Job drawing, mm, ordinate dimensions from the low corner. One solid piece. A direction names the side the tool comes from. Coordinates: 2 decimals unless noted, no trailing zeros. Write each loop counter-clockwise with the first axis right and the second up, starting at its lowest first coordinate (ties: lowest second). Pieces come first, ordered by that corner, then holes. Notation, with made-up numbers: (44, 81) -> (87, 81) arc R3 ccw to (87, 85) -> close; hole circle Ø5 at (62.5, -3.5). An arc over 180 degrees is marked (long way). One line per question, with ' | ' between items. Start each with the question number.
Item 1: 3-axis set-ups, long thin cutter, end or side, ignore diameter. For the marked faces 1 and 2: which of +Z, -Z, +X, -X, +Y, -Y reach the whole face in a straight line?
Item 2: Saw through at D-D (y = 4.5). List the corners of the cut face in (x, z).
Item 3: Pin check, flat tips, straight feed: pin 1 (1 mm diameter, centred on x = 17.5, z = 0.5, fed in from +Y); pin 2 (4 mm diameter, centred on x = 11, y = 8, fed in from +Z); pin 3 (1.7 mm diameter, centred on x = 11.25, y = 19.75, fed in from +Z). Stop position of each tip, or through.
Item 4: Two-plate mould, pull along Y, no slides. Class the marked faces 3, 4 and 5: pulls with the +Y half, pulls with the -Y half, needs draft (parallel to the pull), parting line crosses it, or undercut.
Item 5: Probe probe 1 along Y at (x, z) = (11.25, 1.2) (1 decimal); probe 2 along Y at (x, z) = (12.5, 1.65) (1 decimal); probe 3 along Z at (x, y) = (10.5, 11.75). List the from-to ranges inside material, lowest first. Write a range as [from, to].
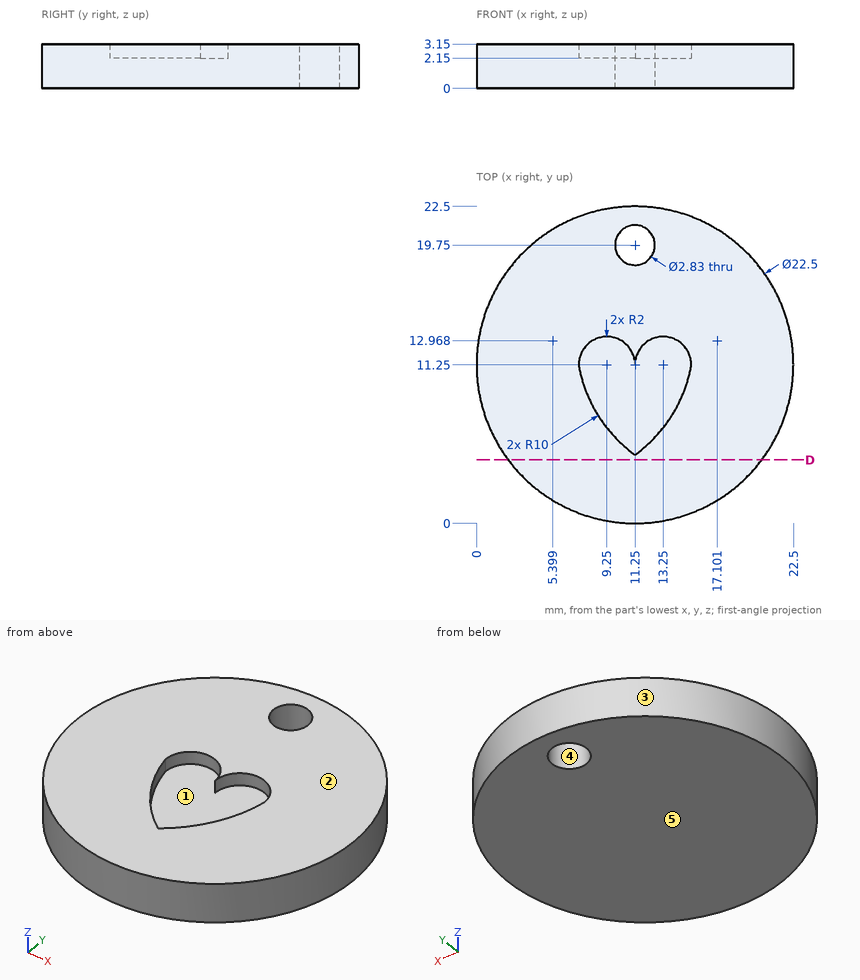
From the geometry:
1) face 1: +Z | face 2: +Z, +X, -X, +Y, -Y
2) outline: (2.25, 0) -> (20.25, 0) -> (20.25, 3.15) -> (2.25, 3.15) -> close
3) pin 1: y = 20.92 | pin 2: z = 2.15 | pin 3: through
4) face 3: parting line crosses it | face 4: undercut | face 5: needs draft
5) probe 1: [0, 18.3], [21.2, 22.5] | probe 2: [0.1, 19.1], [20.4, 22.4] | probe 3: [0, 2.15]
